Design review of the part built by this model. Coordinates are the model's own, in mm. A direction names the side the tool comes from. Coordinates: 2 decimals unless noted, no trailing zeros. Write each loop counter-clockwise with the first axis right and the second up, starting at its lowest first coordinate (ties: lowest second). Pieces come first, ordered by that corner, then holes. Notation, with made-up numbers: (49, 20) - (58, 20) arc R37 ccw to (58, 56) - close; hole circle Ø5 at (48.5, 54). An arc over 180 degrees is marked (long way). Answer as CSV lines item,"result". Start each with the question number.
Q1. Clearance check with flat-ended pins moving along their axes: pin 1 (5 mm diameter, centred on x = -111, z = 98.5, fed in from -Y); pin 2 (5 mm diameter, centred on y = 41, z = 324, fed in from +X); pin 3 (8 mm diameter, centred on y = 37, z = 83.5, fed in from -X); pin 4 (24 mm diameter, centred on x = 0, z = 0, fed in from +Y). State where each tip first meets the part, or that it passes through.
Q2. For line 1 along Y through (x, z) = (-70.5, 0); line 2 along X through (y, z) = (-82, 0); line 3 along X through (y, z) = (-33.5, 320.5), list the stretches that pass through material, from the lowest coordinate up. Write a range as [from, to].
Q3. We need section D-D (z = 176). Write out the cut boundary in (x, y).
Q4. We need section C-C (x = -198.5). Write out the cut boundary in (y, z).
Q5. We need section B-B (z = 313.5). Write out the cut boundary in (x, y) (3 decimals), plus the area to 3 significant figures.
Q6. We need section A-A (x = -49). Write out the cut boundary in (y, z), plus the area to 3 significant figures.
Q7. Mouldability with a two-part tool opening along Z and no side actions: class faces 4 (the face through (-69.86, 1.64, 63.98)), 5 (the face through (-49.86, -91.65, -0.25)), 6 (the face through (-266.343, 34.79, 298.004)), 7 (the face through (40, 5, 70)) as pulls with the +Z half, pulls with the -Z half, needs draft (parallel to the pull), parting line crosses it, or undercut.
Q8. Machinability: for faces 1 (the face through (-263.21, -34.79, 285.33)), 2 (the face through (-60, 26, 73)), 3 (the face through (-0.56, -85.261, -22.846)), which of the approach directions +Z, -Z, +X, -X, +Y, -Y give a long, thin tool a straight path to every point of the face, cutting with its end or side? Answer none if there is none.
from build123d import *

# Parameters (mm, degrees)
F1_ANGLE_BACK  = 105
F1_ANGLE       = 210
F2_R           = 20
F3_DEPTH       = 100.001
F3_DEPTH_BACK  = 100.001
F5_DEPTH       = 20
F7_DEPTH       = 20
F19_DEPTH      = 110.0010001
F19_DEPTH_BACK = 110.0010001


# Not quite as in the source:
# - a feature names something its author has since deleted; it is built from what else it names


with BuildPart() as f1:
    # F0 (on Front) → F1 (revolve)
    with BuildSketch(Plane.XZ, mode=Mode.PRIVATE) as f1_sk:
        with BuildLine():
            Line((40, 69.2820323028), (40, 91.6515138991))
            ThreePointArc((40, 91.6515138991), (0, 100), (-40, 91.6515138991))
            Line((-40, 91.6515138991), (-40, 69.2820323028))
            ThreePointArc((-40, 69.2820323028), (0, 80), (40, 69.2820323028))
        make_face()
    revolve(f1_sk.sketch.rotate(Axis((77.3328692646, 0, 0), (1, 0, 0)), -F1_ANGLE_BACK), axis=Axis((77.3328692646, 0, 0), (1, 0, 0)), revolution_arc=F1_ANGLE)

    # F2 (on Front) → F3 (cut, two sides)
    with BuildSketch(Plane.XZ) as f3_sk:
        Circle(F2_R)
    extrude(amount=-F3_DEPTH, mode=Mode.SUBTRACT)
    extrude(f3_sk.sketch, amount=F3_DEPTH_BACK, mode=Mode.SUBTRACT)

    # F4 (on face) → F5 (join)
    with BuildSketch(Plane(origin=(-40, 0, 0), x_dir=(0, -1, 0), z_dir=(-1, 0, 0))):
        with BuildLine():
            Line((0, 91.6515138991), (0, 69.2820323028))
            ThreePointArc((0, 69.2820323028), (6.7908266825, 68.9484203805), (13.5162539919, 67.950797479))
            Line((13.5162539919, 67.950797479), (17.8803233598, 89.8904557589))
            ThreePointArc((17.8803233598, 89.8904557589), (8.9834192993, 91.2101868088), (0, 91.6515138991))
        make_face()
        with BuildLine():
            ThreePointArc((-57.6059045383, 38.4910348305), (-48.9897948557, 48.9897948557), (-38.4910348305, 57.6059045383))
            Line((-38.4910348305, 57.6059045383), (-50.9188529335, 76.2054487286))
            ThreePointArc((-50.9188529335, 76.2054487286), (-64.8074069841, 64.8074069841), (-76.2054487286, 50.9188529335))
            Line((-76.2054487286, 50.9188529335), (-57.6059045383, 38.4910348305))
        make_face()
        with BuildLine():
            ThreePointArc((-67.950797479, -13.5162539919), (-69.2820323028, 0), (-67.950797479, 13.5162539919))
            Line((-67.950797479, 13.5162539919), (-89.8904557589, 17.8803233598))
            ThreePointArc((-89.8904557589, 17.8803233598), (-91.6515138991, 0), (-89.8904557589, -17.8803233598))
            Line((-89.8904557589, -17.8803233598), (-67.950797479, -13.5162539919))
        make_face()
        with BuildLine():
            Line((50.9188529335, 76.2054487286), (38.4910348305, 57.6059045383))
            ThreePointArc((38.4910348305, 57.6059045383), (48.9897948557, 48.9897948557), (57.6059045383, 38.4910348305))
            Line((57.6059045383, 38.4910348305), (76.2054487286, 50.9188529335))
            ThreePointArc((76.2054487286, 50.9188529335), (64.8074069841, 64.8074069841), (50.9188529335, 76.2054487286))
        make_face()
        with BuildLine():
            ThreePointArc((-13.5162539919, 67.950797479), (-6.7908266825, 68.9484203805), (0, 69.2820323028))
            Line((0, 69.2820323028), (0, 91.6515138991))
            ThreePointArc((0, 91.6515138991), (-8.9834192993, 91.2101868088), (-17.8803233598, 89.8904557589))
            Line((-17.8803233598, 89.8904557589), (-13.5162539919, 67.950797479))
        make_face()
        with BuildLine():
            Line((89.8904557589, 17.8803233598), (67.950797479, 13.5162539919))
            ThreePointArc((67.950797479, 13.5162539919), (68.9484203805, 6.7908266825), (69.2820323028, 0))
            ThreePointArc((69.2820323028, 0), (68.9484203805, -6.7908266825), (67.950797479, -13.5162539919))
            Line((67.950797479, -13.5162539919), (89.8904557589, -17.8803233598))
            ThreePointArc((89.8904557589, -17.8803233598), (91.6515138991, 0), (89.8904557589, 17.8803233598))
        make_face()
    extrude(amount=F5_DEPTH)

    # F6 (on face) → F7 (join)
    with BuildSketch(Plane(origin=(-60, 0, 0), x_dir=(0, -1, 0), z_dir=(-1, 0, 0))):
        with BuildLine():
            Line((61.8192528825, -16.5644188866), (106.2518408918, -28.4700949613))
            ThreePointArc((106.2518408918, -28.4700949613), (0, 110), (-106.2518408918, -28.4700949613))
            Line((-106.2518408918, -28.4700949613), (-61.8192528825, -16.5644188866))
            ThreePointArc((-61.8192528825, -16.5644188866), (0, 64), (61.8192528825, -16.5644188866))
        make_face()
    extrude(amount=F7_DEPTH)

    # F7_face (on face) → F11 section 0
    with BuildSketch(Plane(origin=(-80, 0, 46.9243182834), x_dir=(0, -1, 0), z_dir=(-1, 0, 0))):
        with BuildLine():
            Line((-106.2518408918, -75.3944132447), (-61.8192528825, -63.4887371699))
            ThreePointArc((-61.8192528825, -63.4887371699), (0, 17.0756817166), (61.8192528825, -63.4887371699))
            Line((61.8192528825, -63.4887371699), (106.2518408918, -75.3944132447))
            ThreePointArc((106.2518408918, -75.3944132447), (0, 63.0756817166), (-106.2518408918, -75.3944132447))
        make_face()
    # F9 (on offset) → F11 section 1
    with BuildSketch(Plane(origin=(-180, 0, 0), x_dir=(0, -1, 0), z_dir=(-1, 0, 0))):
        with BuildLine():
            Line((20, 60), (50, 60))
            ThreePointArc((50, 60), (0, 110), (-50, 60))
            Line((-50, 60), (-20, 60))
            ThreePointArc((-20, 60), (0, 80), (20, 60))
        make_face()
    loft()

    # F16 (on face) → F17 (join, up to the next surface of F1)
    with BuildSketch(Plane(origin=(-163.3136094675, 0, 391.9526627219), x_dir=(0.9230769231, 0, 0.3846153846), z_dir=(-0.3846153846, 0, 0.9230769231))):
        Polygon((-143.0769230769, -20), (-143.0769230769, -50), (-23.0769230769, -50), (-23.0769230769, 50), (-143.0769230769, 50), (-143.0769230769, 20), (-63.0769230769, 20), (-63.0769230769, -20), align=None)
    extrude(until=Until.NEXT, dir=(0.3846153846, 0, -0.9230769231))

    # F18 (on Front) → F19 (cut, two sides)
    with BuildSketch(Plane.XZ) as f19_sk:
        with BuildLine():
            Line((-295.3846153846, 336.9230769231), (-272.3076923077, 281.5384615385))
            ThreePointArc((-272.3076923077, 281.5384615385), (-274.8460121427, 288.9650307682), (-276.3932544968, 296.6593818913))
            ThreePointArc((-276.3932544968, 296.6593818913), (-268.9472491257, 334.5066125365), (-240.0000021838, 359.9999990901))
            Line((-240.0000021838, 359.9999990901), (-295.3846153846, 336.9230769231))
        make_face()
        with BuildLine():
            ThreePointArc((-240.0000021838, 359.9999990901), (-194.0780897016, 360.0960709742), (-161.5384615385, 327.6923076923))
            Line((-161.5384615385, 327.6923076923), (-184.6153846154, 383.0769230769))
            Line((-184.6153846154, 383.0769230769), (-240.0000021838, 359.9999990901))
        make_face()
        with BuildLine():
            Line((-216.9230769231, 304.6153846154), (-180, 320))
            ThreePointArc((-180, 320), (-227.3566461545, 343.2306747618), (-256.5698619723, 299.3113827993))
            Line((-256.5698619723, 299.3113827993), (-216.9230769231, 304.6153846154))
        make_face()
        with BuildLine():
            ThreePointArc((-256.5698619723, 299.3113827993), (-255.5383670695, 294.1818153839), (-253.8461538462, 289.2307692308))
            Line((-253.8461538462, 289.2307692308), (-216.9230769231, 304.6153846154))
            Line((-216.9230769231, 304.6153846154), (-256.5698619723, 299.3113827993))
        make_face()
        with BuildLine():
            ThreePointArc((-253.8461538462, 289.2307692308), (-209.0784315175, 265.3921575877), (-176.9230769231, 304.6153846154))
            ThreePointArc((-176.9230769231, 304.6153846154), (-177.6998498954, 312.4600300209), (-180, 320))
            Line((-180, 320), (-216.9230769231, 304.6153846154))
            Line((-216.9230769231, 304.6153846154), (-253.8461538462, 289.2307692308))
        make_face()
        with BuildLine():
            Line((-272.3076923077, 281.5384615385), (-253.8461538462, 289.2307692308))
            ThreePointArc((-253.8461538462, 289.2307692308), (-255.5383670695, 294.1818153839), (-256.5698619723, 299.3113827993))
            Line((-256.5698619723, 299.3113827993), (-276.3932544968, 296.6593818913))
            ThreePointArc((-276.3932544968, 296.6593818913), (-274.8460121427, 288.9650307682), (-272.3076923077, 281.5384615385))
        make_face()
    extrude(amount=-F19_DEPTH, mode=Mode.SUBTRACT)
    extrude(f19_sk.sketch, amount=F19_DEPTH_BACK, mode=Mode.SUBTRACT)


solid = f1.part
Results list:
1,pin 1,"stops at y = -50"
1,pin 2,"stops at x = -158.96"
1,pin 3,"stops at x = -191.46"
1,pin 4,"passes through"
2,line 1,"y = [-110, -64], [64, 110]"
2,line 2,"x = [-110.53, -20], [20, 40]"
2,line 3,"x = [-274.78, -253.63], [-180.21, -158.54]"
3,outline,"(-228.33, -50) - (-98.33, -50) - (-98.33, 50) - (-228.33, 50) - (-228.33, 20) - (-141.67, 20) - (-141.67, -20) - (-228.33, -20) - close"
4,outline,"(-50, 104.4) - (-20, 104.4) - (-20, 269.11) - (-50, 269.11) - close; (-50, 340.12) - (50, 340.12) - (50, 361.72) - (-50, 361.72) - close; (20, 104.4) - (50, 104.4) - (50, 269.11) - (20, 269.11) - close"
5,outline,"(-276.262, -50) - (-255.924, -50) - (-255.924, -20) - (-276.262, -20) - close; (-276.262, 20) - (-255.924, 20) - (-255.924, 50) - (-276.262, 50) - close; (-177.922, -50) - (-155.625, -50) - (-155.625, 50) - (-177.922, 50) - close"
5,area,"3,450 mm2"
6,outline,"(-89.89, -17.88) - (-67.95, -13.52) arc R69.28 cw to (-67.95, 13.52) - (-89.89, 17.88) arc R91.65 ccw to start; (-76.21, 50.92) - (-57.61, 38.49) arc R69.28 cw to (-38.49, 57.61) - (-50.92, 76.21) arc R91.65 ccw to start; (-17.88, 89.89) - (-13.52, 67.95) arc R69.28 cw to (13.52, 67.95) - (17.88, 89.89) arc R91.65 ccw to start; (38.49, 57.61) arc R69.28 cw to (57.61, 38.49) - (76.21, 50.92) arc R91.65 ccw to (50.92, 76.21) - close; (67.95, -13.52) - (89.89, -17.88) arc R91.65 ccw to (89.89, 17.88) - (67.95, 13.52) arc R69.28 cw to start"
6,area,"3,530 mm2"
7,face 4,"undercut"
7,face 5,"parting line crosses it"
7,face 6,"undercut"
7,face 7,"needs draft"
8,face 1,"-X, +Y, -Y"
8,face 2,"none"
8,face 3,"-Z, +X, -X"
